```python
from build123d import *

# Parameters (mm, degrees)
F1_W     = 127
F1_H     = 127
F1_W_2   = 101.6
F1_H_2   = 101.6
F2_DEPTH = 25.4
F3_R     = 5.08


with BuildPart() as f2:
    # F1 (on face) → F2 (new body)
    with BuildSketch(Plane.XY):
        with Locations((8.968271, -6.068526)):
            Rectangle(F1_W, F1_H)
        with Locations((8.968271, -6.068526)):
            Rectangle(F1_W_2, F1_H_2, mode=Mode.SUBTRACT)
    extrude(amount=F2_DEPTH)

    # F3
    f3_edges = [f2.edges().sort_by_distance(p)[0] for p in [
        (8.968271, -56.868526, 25.4),
        (59.768271, -6.068526, 25.4),
        (-41.831729, -6.068526, 25.4),
        (8.968271, 44.731474, 25.4),
    ]]
    fillet(f3_edges, radius=F3_R)


solid = f2.part
```
Part model, mm, in its own coordinate system. A direction names the side the tool comes from. Round coordinates to 2 decimals unless told otherwise and drop trailing zeros. Order: outer loops, then holes, each group sorted by start corner. A loop starts at its lowest first (then second) coordinate and runs counter-clockwise, first axis right, second up. Notation, with made-up numbers: M 1.25,7 L 48.25,7 A31 ccw 48.25,43 Z; hole C 27.25,6.5 d5. An arc over 180 degrees is marked long. Put each result on its own line as item: value. Start each with the question number.
1. Two-plate mould, pull along Y, no slides. Class faces 1 (the face through (61.217, -5.286, 23.872)), 2 (the face through (8, 57.431, 13)), 3 (the face through (-48, -6, 25.4)): +Y half, -Y half, draft (parallel to the pull), parting line (faces both ways), or undercut.
2. Slice it at A-A on x = -16. List the corners of the cut face in (y, z), then the cut area to 3 significant figures.
3. Slice it at B-B on y = -9.5. List the corners of the cut face in (x, z), then the cut area to 3 significant figures.
4. Slice it at C-C on z = 17. List the corners of the cut face in (x, y), then the cut area to 3 significant figures.
5. Drill centre lines: probe 1 along X at (y, z) = (-44, 14.5); probe 2 along Y at (x, z) = (7, 3); probe 3 along Y at (x, z) = (22, 22.5). Where is each one in solid material? Low to high. Write a range as [from, to].
6. Tool access for faces 4 (the face through (9.751, -58.317, 23.872)), 5 (the face through (59.768, -7, 10)), 6 (the face through (8, -69.569, 13)): list every direction of +Z, -Z, +X, -X, +Y, -Y with a clear straight run to the whole face (end or side of a thin tool).
Findings:
1. face 1: undercut
1. face 2: +Y half
1. face 3: draft
2. outline: M -69.57,0 L -56.87,0 L -56.87,20.32 A5.08 ccw -61.95,25.4 L -69.57,25.4 Z; M 44.73,0 L 57.43,0 L 57.43,25.4 L 49.81,25.4 A5.08 ccw 44.73,20.32 Z
2. area: 634 mm2
3. outline: M -54.53,0 L -41.83,0 L -41.83,20.32 A5.08 ccw -46.91,25.4 L -54.53,25.4 Z; M 59.77,0 L 72.47,0 L 72.47,25.4 L 64.85,25.4 A5.08 ccw 59.77,20.32 Z
3. area: 634 mm2
4. outline: M -54.53,-69.57 L 72.47,-69.57 L 72.47,57.43 L -54.53,57.43 Z; hole M -41.83,-56.87 L 59.77,-56.87 L 59.77,44.73 L -41.83,44.73 Z
4. area: 5,810 mm2
5. probe 1: [-54.53, -41.83], [59.77, 72.47]
5. probe 2: [-69.57, -56.87], [44.73, 57.43]
5. probe 3: [-69.57, -57.36], [45.22, 57.43]
6. face 4: +Z
6. face 5: +Z, -Z
6. face 6: +Z, -Z, +X, -X, -Y
